Work out the finished part from the listing and answer in its coordinate system (mm). Face numbers are marked on the shaded views. A direction names the side the tool comes from. Give positions to 0.01 mm unless a question says otherwise; leave off trailing zeros. Write each loop counter-clockwise with the first axis right and the second up, starting at its lowest first coordinate (ties: lowest second). Pieces come first, ordered by that corner, then holes.
1) Given pin 1 Ø1.5 at (x, y) = (27.5, 45.5) entering from +Z; pin 2 Ø5 at (x, y) = (22.5, 10.5) entering from +Z; pin 3 Ø2 at (x, y) = (8.5, 27) entering from +Z, each flat-ended and moving along its own axis, determine where each tip first touches the part or whether it passes through.
2) Find section B-B (x = 39.5). Determine the outline of the cut face in (y, z).
3) A tool of negligible diameter and unlimited length cuts with its end or side. For the marked faces 1 and 2, from which of +Z, -Z, +X, -X, +Y, -Y can it reach the whole face along a straight path? Write none if from no direction.
4) Straight lines are drawn through the part: probe 1 along Y at (x, z) = (21, -23.5); probe 2 along Y at (x, z) = (20.5, -9); probe 3 along Y at (x, z) = (24, -18). For each, find the intervals that lie inside material, in ascending order.
5) Find section C-C (y = 14.5). Determine the outline of the cut face in (x, z).
6) Find section D-D (z = 22). Determine the outline of the cut face in (x, y), plus the area to 3 significant figures.
```python
from build123d import *

# Parameters (mm, degrees)
F1_DEPTH       = 50
F2_DEPTH       = 5
F4_D           = 9.5
F4_CBORE_D     = 18.6
F4_CBORE_DEPTH = 7
F5_T1_DEPTH    = 50
F6_R           = 2
F7_R           = 2
F8_R           = 2
F9_R           = 2
F10_R          = 2
F11_SIZE       = 1
F12_SIZE       = 1
F3_R           = 7.4475
F3_R_2         = 4.7406141581
F13_DEPTH      = 11


# Not quite as in the source:
# - a fillet or chamfer that OpenCascade refuses, or shapes differently, is made with other operations: its cross-section is extruded or revolved along the edge and cut away or added
# - a feature names something its author has since deleted; it is built from what else it names


with BuildPart() as f1:
    # F0 (on Right) → F1 (new body)
    with BuildSketch(Plane.YZ):
        with BuildLine():
            Line((-36.8190155774, -18.3037728071), (-36.8190155774, -43.3037728071))
            Line((-36.8190155774, -43.3037728071), (-30.8190155774, -43.3037728071))
            Line((-30.8190155774, -43.3037728071), (-30.8190155774, -22.0011100173))
            Line((-30.8190155774, -22.0011100173), (-25.8190155774, -22.0011100173))
            Line((-25.8190155774, -22.0011100173), (-25.8190155774, -43.3037728071))
            Line((-25.8190155774, -43.3037728071), (-19.8190155774, -43.3037728071))
            Line((-19.8190155774, -43.3037728071), (-19.8190155774, -18.3037728071))
            ThreePointArc((-19.8190155774, -18.3037728071), (-6.0172669539, 21.0281033399), (30.1809844226, 41.6962271929))
            Line((30.1809844226, 41.6962271929), (54.8554914248, 45.7172599205))
            Line((54.8554914248, 45.7172599205), (53.2470783337, 55.5870627214))
            Line((53.2470783337, 55.5870627214), (28.5725713315, 51.5660299938))
            ThreePointArc((28.5725713315, 51.5660299938), (-16.0298177258, 27.7745861378), (-36.8190155774, -18.3037728071))
        make_face()
    extrude(amount=F1_DEPTH)

    # F2 (add): a face of the model
    f2_faces = [f1.faces().sort_by_distance(p)[0] for p in [
        (25, 40.9098248326, 53.5765463576),
    ]]
    extrude(f2_faces, amount=F2_DEPTH)

    # F4 (through all)
    with Locations(Plane(origin=(0, -8.2509991118, 50.6311062727), x_dir=(1, 0, 0), z_dir=(0, -0.1608413091, 0.9869802801))):
        with Locations((25, 48.9945122253)):
            CounterBoreHole(F4_D / 2, F4_CBORE_D / 2, F4_CBORE_DEPTH)

    # F5: fillet of radius 12 on 1 edges, made by hand

    # F5_s2 → F5_t1 (join)
    with BuildSketch(Plane.YZ):
        with BuildLine():
            ThreePointArc((19.9803220456, 49.6650925191), (24.650251765, 52.1990228082), (27.768364786, 56.5009313942))
            Line((27.768364786, 56.5009313942), (28.5725713315, 51.5660299938))
            ThreePointArc((28.5725713315, 51.5660299938), (24.2497369804, 50.7362893045), (19.9803220456, 49.6650925191))
        make_face()
    extrude(amount=F5_T1_DEPTH)

    # F6
    f6_edges = [f1.edges().sort_by_distance(p)[0] for p in [
        (25, 27.768365, 56.500931),
    ]]
    fillet(f6_edges, radius=F6_R)

    # F7
    f7_edges = [f1.edges().sort_by_distance(p)[0] for p in [
        (25, 52.442872, 60.521964),
    ]]
    fillet(f7_edges, radius=F7_R)

    # F8
    f8_edges = [f1.edges().sort_by_distance(p)[0] for p in [
        (25, 54.855491, 45.71726),
    ]]
    fillet(f8_edges, radius=F8_R)

    # F9
    f9_edges = [f1.edges().sort_by_distance(p)[0] for p in [
        (25, -19.819016, -43.303773),
    ]]
    fillet(f9_edges, radius=F9_R)

    # F10
    f10_edges = [f1.edges().sort_by_distance(p)[0] for p in [
        (25, -36.819016, -43.303773),
    ]]
    fillet(f10_edges, radius=F10_R)

    # F11
    f11_edges = [f1.edges().sort_by_distance(p)[0] for p in [
        (25, -30.819016, -22.00111),
    ]]
    chamfer(f11_edges, length=F11_SIZE)

    # F12
    f12_edges = [f1.edges().sort_by_distance(p)[0] for p in [
        (25, -25.819016, -22.00111),
    ]]
    chamfer(f12_edges, length=F12_SIZE)

    # F3 (on face) → F13 (cut)
    with BuildSketch(Plane(origin=(0, -8.2509991118, 50.6311062727), x_dir=(1, 0, 0), z_dir=(0, -0.1608413091, 0.9869802801))):
        with Locations((25, 48.9945122253)):
            Circle(F3_R)
        with Locations((25, 48.9945122253)):
            Circle(F3_R_2, mode=Mode.SUBTRACT)
    extrude(amount=-F13_DEPTH, mode=Mode.SUBTRACT)


solid = f1.part
```
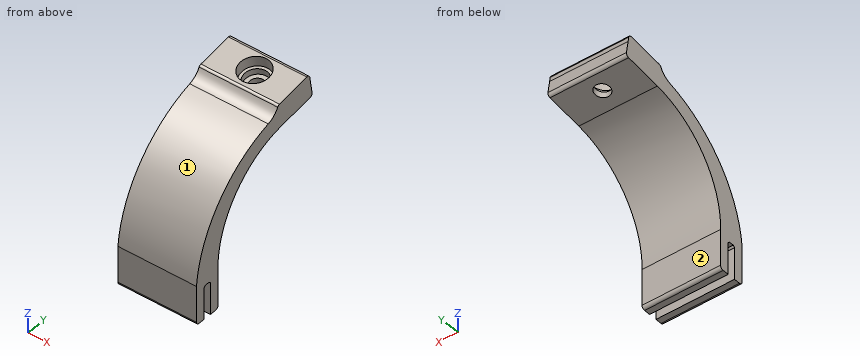
Results:
1. pin 1: stops at z = 48.37
1. pin 2: stops at z = 47.35
1. pin 3: stops at z = 56.35
2. outline: (-36.82, -41.3) arc R2 ccw to (-34.82, -43.3) - (-30.82, -43.3) - (-30.82, -23) - (-29.82, -22) - (-26.82, -22) - (-25.82, -23) - (-25.82, -43.3) - (-21.82, -43.3) arc R2 ccw to (-19.82, -41.3) - (-19.82, -18.3) arc R59.6 cw to (30.18, 41.7) - (52.88, 45.4) arc R2 ccw to (54.53, 47.69) - (52.76, 58.55) arc R2 ccw to (50.47, 60.2) - (28.8, 56.67) arc R2 ccw to (27.35, 55.63) arc R12 cw to (19.98, 49.67) arc R78.35 ccw to (-36.82, -18.3) - close
3. face 1: +Z, +X, -X, -Y
3. face 2: -Z, +X, -X, +Y
4. probe 1: y = -36.82 to -30.82, -25.82 to -19.82
4. probe 2: y = -35.36 to -19.27
4. probe 3: y = -36.79 to -19.82
5. outline: (0, 36.85) - (50, 36.85) - (50, 47.91) - (0, 47.91) - close
6. outline: (0, -20.93) - (50, -20.93) - (50, -5.19) - (0, -5.19) - close
6. area: 787 mm2
